```python
from build123d import *

# Parameters (mm, degrees)
F1_DEPTH  = 4
F3_DEPTH  = 3
F2_W      = 5
F2_H      = 8
F4_DEPTH  = 2.5
F6_R      = 2.5
F7_DEPTH  = 2
F8_R      = 1.25
F9_DEPTH  = 10
F10_R     = 2.5
F10_R_2   = 1.5
F12_R     = 2.5
F13_DEPTH = 2


with BuildPart() as f1:
    # F0 (on Right) → F1 (new body)
    with BuildSketch(Plane.YZ):
        Polygon((-8, 0), (0, 0), (0, 9), (-24, 9), (-24, 7.5), align=None)
    extrude(amount=F1_DEPTH)

    # F2 (on face) → F3 (cut)
    with BuildSketch(Plane(origin=(0, 0, 0), x_dir=(0, -1, 0), z_dir=(-1, 0, 0))):
        Polygon((23, 9), (8, 9), (8, 1.6566184732), (23, 8.6878684732), align=None)
    extrude(amount=-F3_DEPTH, mode=Mode.SUBTRACT)

    # F2 (on face) → F4 (cut)
    with BuildSketch(Plane(origin=(0, 0, 0), x_dir=(0, -1, 0), z_dir=(-1, 0, 0))):
        with Locations((4, 4)):
            Rectangle(F2_W, F2_H)
    extrude(amount=-F4_DEPTH, mode=Mode.SUBTRACT)

    # F5: F1 across face


with BuildPart() as f1_1:
    add(f1.part)
    add(f1.part.mirror(Plane(origin=(0, -9.4545581434, 4.8825876623), x_dir=(0, 1, 0), z_dir=(-1, 0, 0))))

    # F6 (on face) → F7 (join)
    with BuildSketch(Plane.XY.offset(9)):
        with Locations((0, -4)):
            Circle(F6_R)
    extrude(amount=F7_DEPTH)

    # F8 (on face) → F9 (cut)
    with BuildSketch(Plane(origin=(0, 0, 0), x_dir=(1, 0, 0), z_dir=(0, 0, -1))):
        with Locations((0, 4)):
            Circle(F8_R)
    extrude(amount=-F9_DEPTH, mode=Mode.SUBTRACT)

    # F10 (on face) → F11 (join, up to the next surface of F1)
    with BuildSketch(Plane.XY.offset(11)):
        with Locations((0, -12)):
            Circle(F10_R)
        with Locations((0, -12)):
            Circle(F10_R_2, mode=Mode.SUBTRACT)
        with Locations((0, -20)):
            Circle(F10_R)
        with Locations((0, -20)):
            Circle(F10_R_2, mode=Mode.SUBTRACT)
    extrude(until=Until.NEXT, dir=(0, 0, -1))

    # F12 (on face) → F13 (cut)
    with BuildSketch(Plane(origin=(0, 0, 0), x_dir=(1, 0, 0), z_dir=(0, 0, -1))):
        with Locations((0, 12)):
            Circle(F12_R)
    extrude(amount=-F13_DEPTH, mode=Mode.SUBTRACT)


solid = f1_1.part
```
Work out the finished part from the listing and answer in its coordinate system (mm). A direction names the side the tool comes from. Give positions to 0.01 mm unless a question says otherwise; leave off trailing zeros. Order: outer loops, then holes, each group sorted by start corner. A loop starts at its lowest first (then second) coordinate and runs counter-clockwise, first axis right, second up.
1. The mould has two halves that part along X. Classify faces 1 (the flat face through (-4, -10, 6)), 2 (the flat face through (0, -1, 0)), 3 (the cylindrical face through (-0.33, -9.52, 7.69)), 4 (the flat face through (0, -6.5, 4)): released by +X, released by -X, zero draft, split by the parting line, or undercut.
Result sheet:
face 1: released by -X
face 2: zero draft
face 3: undercut
face 4: undercut
2. For faces 5 (the flat face through (0, -14, 11)), 6 (the flat face through (0, -1.5, 4)), 7 (the flat face through (0, -11, 2)), 8 (the cylindrical face through (-0.195, -18.513, 9.257)), determine the directions among +Z, -Z, +X, -X, +Y, -Y from which every point of the face is accessible in a straight line to the end or side of a thin tool.
Result sheet:
face 5: +Z, +X, -X, +Y, -Y
face 6: -Z
face 7: -Z, -Y
face 8: +Z
3. Section B-B, the plane y = -4 is taken. Determine the outline of the cut face in (x, z), and give its area (3 significant figures).
Result sheet:
outline: (-4, 0) - (-2.5, 0) - (-2.5, 8) - (-1.25, 8) - (-1.25, 10) - (1.25, 10) - (1.25, 8) - (2.5, 8) - (2.5, 0) - (4, 0) - (4, 9) - (2.5, 9) - (2.5, 11) - (-2.5, 11) - (-2.5, 9) - (-4, 9) - close
area: 37.0 mm2
4. Section D-D, the plane x = 1.75 is taken. Determine the outline of the cut face in (y, z).
Result sheet:
outline: (-24, 7.5) - (-12.27, 2) - (-10.21, 2) - (-10.21, 1.04) - (-8, 0) - (-6.5, 0) - (-6.5, 8) - (-1.5, 8) - (-1.5, 0) - (0, 0) - (0, 9) - (-2.21, 9) - (-2.21, 11) - (-5.79, 11) - (-5.79, 9) - (-8, 9) - (-8, 1.66) - (-10.21, 2.69) - (-10.21, 11) - (-13.79, 11) - (-13.79, 4.37) - (-18.21, 6.44) - (-18.21, 11) - (-21.79, 11) - (-21.79, 8.12) - (-23, 8.69) - (-23, 9) - (-24, 9) - close
5. Section A-A, the plane z = 5 is taken. Determine the outline of the cut face in (x, y).
Result sheet:
outline: (-4, -18.67) - (4, -18.67) - (4, 0) - (-4, 0) - close; circle Ø5 at (0, -12); hole (-3, -15.13) - (3, -15.13) - (3, -8) - (-3, -8) - close; hole (-2.5, -6.5) - (2.5, -6.5) - (2.5, -1.5) - (-2.5, -1.5) - close; hole circle Ø3 at (0, -12)
6. Each of these flat-tipped pins is pushed along its axis until it touches: P1, Ø2.5, axis at x = 0, y = -12, coming from the -Z side; P2, Ø3, axis at y = -18.5, z = 1.5, coming from the +X side; P3, Ø1.8, axis at x = -0.5, z = 6, coming from the -Y side; P4, Ø1.2, axis at x = -0.5, y = -4.5, coming from the -Z side. Where does it stop, or does it pass through?
Result sheet:
P1: stops at z = 2
P2: passes through
P3: stops at y = -22.72
P4: stops at z = 8
7. Straight lines are drawn through the part: L1, parallel to X at y = -20, z = 8.75; L2, parallel to X at y = -6, z = 3.5; L3, parallel to Y at x = 0, z = 8.05. For each, find the intervals that lie inside material, in ascending order.
Result sheet:
L1: x = -4 to -3, -2.5 to -1.5, 1.5 to 2.5, 3 to 4
L2: x = -4 to -2.5, 2.5 to 4
L3: y = -24 to -21.5, -18.5 to -17.5, -14.5 to -13.5, -10.5 to -9.5, -8 to -5.25, -2.75 to 0
8. Section C-C, the plane x = -3.25 is taken. Determine the outline of the cut face in (y, z).
Result sheet:
outline: (-24, 7.5) - (-8, 0) - (0, 0) - (0, 9) - (-24, 9) - close
